from build123d import *

# Parameters (mm, degrees)
BOSS_EXTRUDE1_DEPTH = 50.8
FILLET2_R           = 12.7
CHAMFER1_SIZE       = 5.08
SHELL1_T            = -2.54
CUT_EXTRUDE1_DEPTH  = 204.596488182


with BuildPart() as part:
    # Sketch1 → Boss-Extrude1 (new, symmetric)
    with BuildSketch(Plane.XY):
        Polygon((0, 0), (0, 82.55), (-25.4, 107.95), (-25.4, 152.4), (-88.9, 152.4), (-88.9, 65.828865162), (-63.5, 40.428865162), (-63.5, 0), align=None)
    extrude(amount=BOSS_EXTRUDE1_DEPTH, both=True)

    # Fillet2
    fillet2_edges = [part.edges().sort_by_distance(p)[0] for p in [
        (-25.4, 107.95, 0),
        (0, 82.55, 0),
        (-57.15, 152.4, 50.8),
        (-57.15, 152.4, -50.8),
    ]]
    fillet(fillet2_edges, radius=FILLET2_R)

    # Chamfer1
    chamfer1_edges = [part.edges().sort_by_distance(p)[0] for p in [
        (0, 38.644743879, -50.8),
        (-12.7, 95.25, -50.8),
        (-12.7, 95.25, 50.8),
        (-25.4, 126.455256121, -50.8),
        (-0.966729937, 82.149567349, -50.8),
        (-25.4, 126.455256121, 50.8),
        (-0.966729937, 82.149567349, 50.8),
        (-25.4, 152.4, 0),
        (-25.4, 148.680256121, 47.080256121),
        (-25.4, 148.680256121, -47.080256121),
        (-24.433270063, 108.350432651, -50.8),
        (-24.433270063, 108.350432651, 50.8),
        (0, 38.644743879, 50.8),
    ]]
    chamfer(chamfer1_edges, length=CHAMFER1_SIZE)

    # Shell1
    shell1_openings = [part.faces().sort_by_distance(p)[0] for p in [
        (-63.5, 20.214432581, 0),
        (-76.2, 53.128865162, 0),
        (-88.9, 108.793553587, 0),
        (-31.870709505, 0, 0),
    ]]
    offset(amount=SHELL1_T, openings=shell1_openings, kind=Kind.INTERSECTION)

    # Sketch2 → Cut-Extrude1 (cut, through all)
    with BuildSketch(Plane.XY.offset(50.8)):
        with BuildLine():
            Line((-75.481467356, 133.437271175), (-48.129261469, 133.437271175))
            ThreePointArc((-48.129261469, 133.437271175), (-46.721269062, 132.496480726), (-47.051630735, 130.835640441))
            Line((-47.051630735, 130.835640441), (-50.44090191, 127.446369265))
            ThreePointArc((-50.44090191, 127.446369265), (-50.935323093, 127.116007592), (-51.518532644, 127))
            Line((-51.518532644, 127), (-78.870738531, 127))
            ThreePointArc((-78.870738531, 127), (-80.278730938, 127.940790449), (-79.948369265, 129.601630735))
            Line((-79.948369265, 129.601630735), (-76.55909809, 132.99090191))
            ThreePointArc((-76.55909809, 132.99090191), (-76.064676907, 133.321263583), (-75.481467356, 133.437271175))
        make_face()
        with BuildLine():
            Line((-75.481467356, 123.277271175), (-48.129261469, 123.277271175))
            ThreePointArc((-48.129261469, 123.277271175), (-46.721269062, 122.336480726), (-47.051630735, 120.675640441))
            Line((-47.051630735, 120.675640441), (-50.44090191, 117.286369265))
            ThreePointArc((-50.44090191, 117.286369265), (-50.935323093, 116.956007592), (-51.518532644, 116.84))
            Line((-51.518532644, 116.84), (-78.870738531, 116.84))
            ThreePointArc((-78.870738531, 116.84), (-80.278730938, 117.780790449), (-79.948369265, 119.441630735))
            Line((-79.948369265, 119.441630735), (-76.55909809, 122.83090191))
            ThreePointArc((-76.55909809, 122.83090191), (-76.064676907, 123.161263583), (-75.481467356, 123.277271175))
        make_face()
        with BuildLine():
            Line((-75.481467356, 113.117271175), (-48.129261469, 113.117271175))
            ThreePointArc((-48.129261469, 113.117271175), (-46.721269062, 112.176480726), (-47.051630735, 110.515640441))
            Line((-47.051630735, 110.515640441), (-50.44090191, 107.126369265))
            ThreePointArc((-50.44090191, 107.126369265), (-50.935323093, 106.796007592), (-51.518532644, 106.68))
            Line((-51.518532644, 106.68), (-78.870738531, 106.68))
            ThreePointArc((-78.870738531, 106.68), (-80.278730938, 107.620790449), (-79.948369265, 109.281630735))
            Line((-79.948369265, 109.281630735), (-76.55909809, 112.67090191))
            ThreePointArc((-76.55909809, 112.67090191), (-76.064676907, 113.001263583), (-75.481467356, 113.117271175))
        make_face()
        with BuildLine():
            Line((-75.481467356, 102.957271175), (-48.129261469, 102.957271175))
            ThreePointArc((-48.129261469, 102.957271175), (-46.721269062, 102.016480726), (-47.051630735, 100.355640441))
            Line((-47.051630735, 100.355640441), (-50.44090191, 96.966369265))
            ThreePointArc((-50.44090191, 96.966369265), (-50.935323093, 96.636007592), (-51.518532644, 96.52))
            Line((-51.518532644, 96.52), (-78.870738531, 96.52))
            ThreePointArc((-78.870738531, 96.52), (-80.278730938, 97.460790449), (-79.948369265, 99.121630735))
            Line((-79.948369265, 99.121630735), (-76.55909809, 102.51090191))
            ThreePointArc((-76.55909809, 102.51090191), (-76.064676907, 102.841263583), (-75.481467356, 102.957271175))
        make_face()
        with BuildLine():
            Line((-75.481467356, 92.797271175), (-48.129261469, 92.797271175))
            ThreePointArc((-48.129261469, 92.797271175), (-46.721269062, 91.856480726), (-47.051630735, 90.195640441))
            Line((-47.051630735, 90.195640441), (-50.44090191, 86.806369265))
            ThreePointArc((-50.44090191, 86.806369265), (-50.935323093, 86.476007592), (-51.518532644, 86.36))
            Line((-51.518532644, 86.36), (-78.870738531, 86.36))
            ThreePointArc((-78.870738531, 86.36), (-80.278730938, 87.300790449), (-79.948369265, 88.961630735))
            Line((-79.948369265, 88.961630735), (-76.55909809, 92.35090191))
            ThreePointArc((-76.55909809, 92.35090191), (-76.064676907, 92.681263583), (-75.481467356, 92.797271175))
        make_face()
        with BuildLine():
            Line((-75.481467356, 82.637271175), (-48.129261469, 82.637271175))
            ThreePointArc((-48.129261469, 82.637271175), (-46.721269062, 81.696480726), (-47.051630735, 80.035640441))
            Line((-47.051630735, 80.035640441), (-50.44090191, 76.646369265))
            ThreePointArc((-50.44090191, 76.646369265), (-50.935323093, 76.316007592), (-51.518532644, 76.2))
            Line((-51.518532644, 76.2), (-78.870738531, 76.2))
            ThreePointArc((-78.870738531, 76.2), (-80.278730938, 77.140790449), (-79.948369265, 78.801630735))
            Line((-79.948369265, 78.801630735), (-76.55909809, 82.19090191))
            ThreePointArc((-76.55909809, 82.19090191), (-76.064676907, 82.521263583), (-75.481467356, 82.637271175))
        make_face()
    extrude(amount=-CUT_EXTRUDE1_DEPTH, mode=Mode.SUBTRACT)


solid = part.part
Can you work these out from the model? Positions are in its coordinate system, mm. A direction names the side the tool comes from. Round coordinates to 2 decimals unless told otherwise and drop trailing zeros. Order: outer loops, then holes, each group sorted by start corner. A loop starts at its lowest first (then second) coordinate and runs counter-clockwise, first axis right, second up. Notation, with made-up numbers: (89.25, 54) - (142.25, 54) arc R17 cw to (142.25, 85) - close; hole circle Ø11 at (67, 40). An arc over 180 degrees is marked (long way). Answer in a Markdown table with one row per item.
(1) Suppose I cut it at B-B, the plane x = -39. Please give me the cut outline in (y, z), plus the area to 3 significant figures.
From the geometry:
| item | result |
|---|---|
| outline | (0, -50.8) - (139.7, -50.8) arc R12.7 ccw to (152.4, -38.1) - (152.4, 38.1) arc R12.7 ccw to (139.7, 50.8) - (0, 50.8) - (0, 48.26) - (139.7, 48.26) arc R10.16 cw to (149.86, 38.1) - (149.86, -38.1) arc R10.16 cw to (139.7, -48.26) - (0, -48.26) - close |
| area | 994 mm2 |
(2) Suppose I cut it at A-A, the plane z = -5.5. Please give me the cut outline in (x, y).
From the geometry:
| item | result |
|---|---|
| outline | (-88.9, 149.86) - (-31.53, 149.86) - (-27.94, 146.27) - (-27.94, 113.21) arc R15.24 ccw to (-23.48, 102.43) - (-5.52, 84.47) arc R10.16 cw to (-2.54, 77.29) - (-2.54, 0) - (0, 0) - (0, 77.29) arc R12.7 ccw to (-3.72, 86.27) - (-21.68, 104.23) arc R12.7 cw to (-25.4, 113.21) - (-25.4, 147.32) - (-30.48, 152.4) - (-88.9, 152.4) - close |
(3) Which directions (+Z, -Z, +X, -X, +Y, -Y) give clear straight access to the entire face, cutting with the end or side of a thin tool? Please do faces 4 (the face through (-26.812, 107.456, 0.625)), 5 (the face through (-14.4, 93.3, -48.3)), 6 (the face through (-78.28, 90.63, 49.55)).
From the geometry:
| item | result |
|---|---|
| face 4 | -X, -Y |
| face 5 | -Z, +X, +Y |
| face 6 | +Z, -Z |
(4) Suppose I cut it at C-C, the plane y = 17. Please give me the cut outline in (x, z), plus the area to 3 significant figures.
From the geometry:
| item | result |
|---|---|
| outline | (-63.5, -50.8) - (-5.08, -50.8) - (0, -45.72) - (0, 45.72) - (-5.08, 50.8) - (-63.5, 50.8) - (-63.5, 48.26) - (-6.13, 48.26) - (-2.54, 44.67) - (-2.54, -44.67) - (-6.13, -48.26) - (-63.5, -48.26) - close |
| area | 555 mm2 |
(5) Please list where these lines run through material, in increasing order: L1, parallel to Z at x = -35.5, y = 126.5; L2, parallel to X at y = 14.5, z = -40; L3, parallel to Z at x = -5, y = 54. Write a range as from..to.
From the geometry:
| item | result |
|---|---|
| L1 | z = -50.8..-48.26, 48.26..50.8 |
| L2 | x = -2.54..0 |
| L3 | z = -50.72..-47.13, 47.13..50.72 |
(6) For P1, Ø1, axis at y = 68, z = -28, coming from the -X side; P2, Ø3, axis at x = -68.5, z = 49, coming from the +Y side; P3, Ø1.3, axis at y = 23.5, z = 50, coming from the -X side; P4, Ø3, axis at x = -55.5, z = -49.5, coming from the -Y side, each with a flat end and sliding along its axis, tell me the tip position at first contact or that it passes through.
From the geometry:
| item | result |
|---|---|
| P1 | stops at x = -2.54 |
| P2 | stops at y = 148.24 |
| P3 | stops at x = -63.5 |
| P4 | stops at y = 0 |
(7) If we mould it in two halves opening along X, with no side actions, what happens to faces 1 (the face through (-29.76, 126.27, -46.49)), 2 (the face through (-27.4, 146.4, -45)), 3 (the face through (-78.28, 110.95, -49.51))? For each: released by +X, released by -X, zero draft, split by the parting line, or undercut.
From the geometry:
| item | result |
|---|---|
| face 1 | released by -X |
| face 2 | released by +X |
| face 3 | undercut |
